Autodesk Inventor part; units mm, degrees
ref_plane "YZ Plane" through (0, 0, 0) normal (1, 0, 0) x (0, 1, 0)
ref_plane "XZ Plane" through (0, 0, 0) normal (0, 1, 0) x (-1, 0, 0)
ref_plane "XY Plane" through (0, 0, 0) normal (0, 0, 1) x (1, 0, 0)
sketch "Sketch1" plane through (0, 0, 0) normal (0, 0, 1) x (1, 0, 0)
  line L0 (0, 0) -> (25.4, 0)
  line L1 (25.4, 0) -> (25.4, 25.4)
  line L2 (25.4, 25.4) -> (0, 25.4)
  line L3 (0, 25.4) -> (0, 0)
  line L4 (1.5875, 23.8125) -> (23.8125, 23.8125)
  line L5 (23.8125, 23.8125) -> (23.8125, 1.5875)
  line L6 (23.8125, 1.5875) -> (1.5875, 1.5875)
  line L7 (1.5875, 1.5875) -> (1.5875, 23.8125)
  dimension "d0" = 25.4
  dimension "d1" = 25.4
  dimension "d2" = 1.5875
extrude "Extrusion1" add sketch "Sketch1" along normal blind 444.5
sketch "Sketch2" plane through (0, 25.4, 0) normal (0, 1, 0) x (1, 0, 0)
  line L0 (25.4, 0) -> (0, 0)
  line L1 (25.4, -444.5) -> (0, -444.5)
  circle A0 centre (12.7, -381) radius 3.3782
  circle A1 centre (12.7, -431.8) radius 3.3782
  circle A2 centre (13.4937, -237.4032) radius 3.3782
  circle A3 centre (13.4937, -303.4032) radius 3.3782
  line L2 (28.0987, -227.8782) -> (28.0987, -312.9282) construction
  line L3 (0.7937, -312.9282) -> (28.0987, -312.9282) construction
  line L4 (0.7937, -227.8782) -> (0.7937, -312.9282)
  line L5 (28.0987, -227.8782) -> (0.7937, -227.8782) construction
  circle A4 centre (12.7, -12.7) radius 3.3782
  circle A5 centre (12.7, -63.5) radius 3.3782
  line L6 (12.7, 0) -> (12.7, -444.5) construction
extrude "Extrusion2" cut sketch "Sketch2" against normal blind 25.4
sketch "Sketch3" plane through (0, 0, 0) normal (-1, 0, 0) x (0, 0, 1)
  circle A0 centre (422.275, 12.7) radius 3.3782
  circle A1 centre (390.525, 12.7) radius 3.3782
  circle A2 centre (305.6657, 12.7) radius 3.3782
  circle A3 centre (235.8157, 12.7) radius 3.3782
  circle A4 centre (53.975, 12.7) radius 3.3782
  circle A5 centre (22.225, 12.7) radius 3.3782
extrude "Extrusion3" cut sketch "Sketch3" against normal blind 25.4
properties part number "Rebuild Shooter Tower Motor Mount Tube" material "Aluminum 6061"
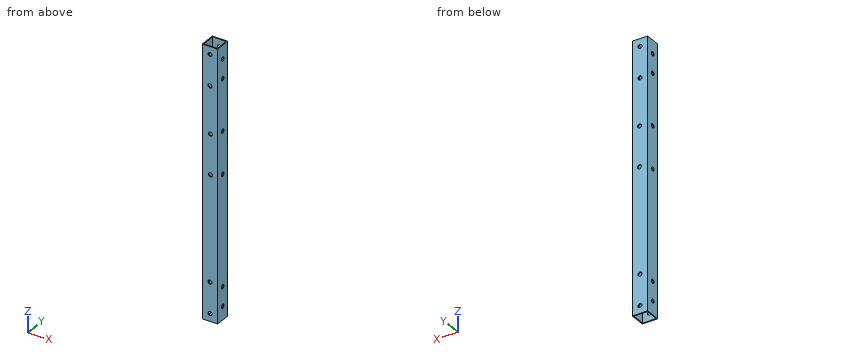
Here's how the part is built. I have some questions about the finished solid (model axes, mm). Coordinates: 2 decimals unless noted, no trailing zeros. Loops run counter-clockwise (first coordinate to the right, second up) from the corner with the lowest first, then second, coordinate; pieces in that order, holes last. Notation, with made-up numbers: (37.5, -30.75) -> (72.5, -30.75) arc R19 cw to (72.5, -2.75) -> close; hole circle Ø6 at (-21, 89.25). An arc over 180 degrees is marked (long way). Use one line per item in the form item = value. Start each with the question number.
(1) If we section it at A-A (y = 5.5): Please give me the cut outline in (x, z), then the cut area to 3 significant figures.
(2) Will this pin go through, and if not, where does the flat tip stop? pin 1 (6 mm diameter, centred on y = 12.7, z = 235.82, fed in from +X).
(3) If we section it at B-B (z = 102): Please give me the cut outline in (x, y), then the cut area to 3 significant figures.
(4) Please list where this line runs through material, in increasing order: line 1 along X through (y, z) = (20.75, 106.5).
Verdict:
q1.outline = (0, 0) -> (1.59, 0) -> (1.59, 444.5) -> (0, 444.5) -> close; (23.81, 0) -> (25.4, 0) -> (25.4, 444.5) -> (23.81, 444.5) -> close
q1.area = 1,410 mm²
q2.pin_1 = through
q3.outline = (0, 0) -> (25.4, 0) -> (25.4, 25.4) -> (0, 25.4) -> close; hole (1.59, 1.59) -> (23.81, 1.59) -> (23.81, 23.81) -> (1.59, 23.81) -> close
q3.area = 151 mm²
q4.line_1 = 0 to 1.59, 23.81 to 25.4
